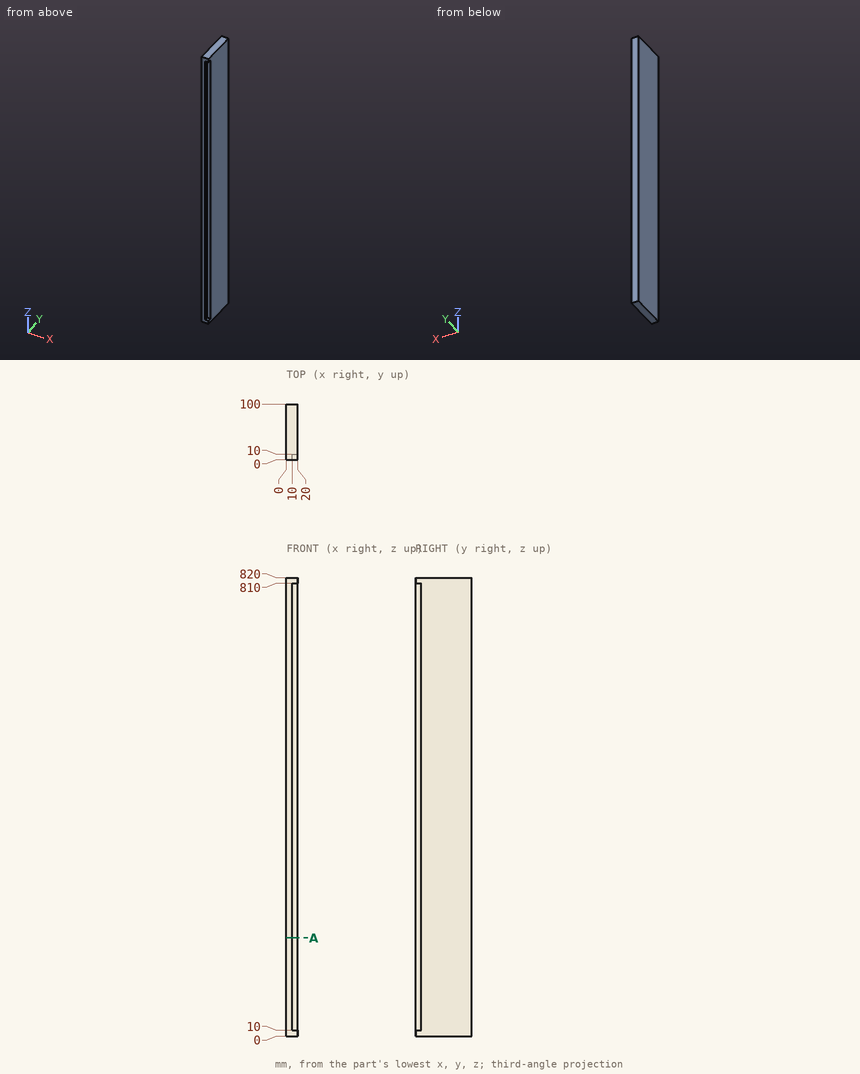
Input: dimensioned drawing with shaded views. Units: mm. Origin: part minimum x, y, z. Coordinates: 2 decimals unless noted, no trailing zeros. Order: outer loops, then holes, each group sorted by start corner. A loop starts at its lowest first (then second) coordinate and runs counter-clockwise, first axis right, second up.
(1) Section query A-A (z = 175.5). Return the cut outline in (x, y), plus the area to 3 significant figures.
(2) Material intervals for probe 1 along Z at (x, y) = (17.25, 4.5); probe 2 along Y at (x, z) = (14.5, 541); probe 3 along X at (y, z) = (7, 101.5), sorted ascending.
(3) First-contact query: pin 1 (3 mm diameter, centred on x = 13, z = 494, fed in from -Y); pin 2 (8 mm diameter, centred on y = 5, z = 570.5, fed in from +X). Flat tips, straight axial feed; report the tip coordinate or a pass-through.
Solution:
1. outline: (0, 0) - (10, 0) - (10, 10) - (20, 10) - (20, 100) - (0, 100) - close
1. area: 1,900 mm2
2. probe 1: z = 0 to 10, 810 to 820
2. probe 2: y = 10 to 100
2. probe 3: x = 0 to 10
3. pin 1: stops at y = 10
3. pin 2: stops at x = 10
